from build123d import *
from build123d.topology import SkipClean

# Parameters (mm, degrees)
SKETCH2_W               = 173
SKETCH2_H               = 29.8
BOSS_EXTRUDE1_DEPTH     = 14
SKETCH4_W               = 173
SKETCH4_H               = 29.8
SKETCH4_R               = 1
BOSS_EXTRUDE3_DEPTH     = 2
BOSS_EXTRUDE4_START     = 5.5
SKETCH5_R               = 1
BOSS_EXTRUDE4_DEPTH     = 5.5
CUT_EXTRUDE1_DEPTH      = 91.874033815
CUT_EXTRUDE1_DEPTH_BACK = 91.874033815


with BuildPart() as part:
    # Sketch2 → Boss-Extrude1 (new body)
    with BuildSketch(Plane(origin=(0, 0, 0), x_dir=(1, 0, 0), z_dir=(0, 1, 0))):
        with Locations((0, 7.9)):
            Rectangle(SKETCH2_W, SKETCH2_H)
        with BuildLine():
            Line((-81.5, 0), (81.5, 0))
            add(Edge.make_bspline(
                [(-81.5, 0), (-74.436091259, 13.881927863), (-43.259356961, 16.362188276), (0, 18.555927536), (43.259356961, 16.362188276), (74.436091259, 13.881927863), (81.5, 0)],
                knots=[0, 0, 0, 0, 0.237125688, 0.5, 0.762874312, 1, 1, 1, 1], degree=3))
        make_face(mode=Mode.SUBTRACT)
    extrude(amount=BOSS_EXTRUDE1_DEPTH)

    # Sketch4 → Boss-Extrude3 (add)
    with BuildSketch(Plane(origin=(0, 14, 0), x_dir=(1, 0, 0), z_dir=(0, 1, 0))):
        with Locations((0, 7.9)):
            Rectangle(SKETCH4_W, SKETCH4_H)
        with Locations(Location((0, 12.8, 0), (0, 0, 270))):
            Circle(SKETCH4_R, mode=Mode.SUBTRACT)
    extrude(amount=BOSS_EXTRUDE3_DEPTH)

    # Sketch5 → Boss-Extrude4 (add)
    with SkipClean():  # the faces are left unmerged after this step: merging them gives an invalid solid
        with BuildSketch(Plane.XZ.offset(-14).offset(BOSS_EXTRUDE4_START)):
            Polygon((0, -9.8), (-7.931348641, -17.731348641), (-7.931348641, -22.8), (7.931348641, -22.8), (7.931348641, -17.731348641), align=None)
            with Locations(Location((0, -12.8, 0), (0, 0, 270))):
                Circle(SKETCH5_R, mode=Mode.SUBTRACT)
        extrude(amount=-BOSS_EXTRUDE4_DEPTH)

    # Sketch3 → Cut-Extrude1 (cut, two sides: drawn at the far end of the back side and taken through both)
    with SkipClean():  # the faces are left unmerged after this step: merging them gives an invalid solid
        with BuildSketch(Plane(origin=(0, 0, 0), x_dir=(0, 0, -1), z_dir=(1, 0, 0)).offset(-CUT_EXTRUDE1_DEPTH_BACK)):
            Polygon((-48.86878806, -37), (4.996225752, 22.823158451), (1.280501625, 26.168811483), (-52.584512187, -33.654346968), align=None)
        extrude(amount=CUT_EXTRUDE1_DEPTH + CUT_EXTRUDE1_DEPTH_BACK, mode=Mode.SUBTRACT)


solid = part.part
Work out the finished part from the listing and answer in its coordinate system (mm). A direction names the side the tool comes from. Give positions to 0.01 mm unless a question says otherwise; leave off trailing zeros. One line per item, written item: value. Start each with the question number.
1. Find section A-A (y = 11). State how many separate pieces and enclosed holes the cut face has, then the cut area to 3 significant figures.
2. Consider probe 1 along Z at (x, y) = (0, 2); probe 2 along X at (y, z) = (15.35, -12.8); probe 3 along Z at (x, y) = (28.5, 8.5). Determine where each line is inside the solid, lowest interval first.
3. Given pin 1 (6 mm diameter, centred on x = -18.5, y = 13, fed in from +Z); pin 2 (8 mm diameter, centred on x = -55.5, z = -5, fed in from -Y); pin 3 (4 mm diameter, centred on x = 53, z = 2, fed in from +Y), each flat-ended and moving along its own axis, determine where each tip first touches the part or whether it passes through.
4. For faces 5 (the flat face through (-1, 16, -11)), 6 (the flat face through (-3.9, 11.2, -13.7)), determine the directions among +Z, -Z, +X, -X, +Y, -Y from which every point of the face is accessible in a straight line to the end or side of a thin tool.
5. For a pull along Z with two mould halves and no side action, classify faces 1 (the flat face through (-86.5, 8, -8)), 2 (the flat face through (4, 11.2, -13.8)), 3 (the flat face through (0, 8.5, -16)), 4 (the flat face through (-1, 5, 7)) as +Z half, -Z half, draft (parallel to the pull), parting line (faces both ways), or undercut.
Geometry results:
1. separate pieces: 1
1. enclosed holes: 2
1. area: 2,550 mm2
2. probe 1: -22.8 to -17.8, 0 to 7
2. probe 2: -86.5 to -1, 1 to 86.5
2. probe 3: -22.8 to -17.01, 0 to 7
3. pin 1: z = 6.55
3. pin 2: y = 14
3. pin 3: y = 16
4. face 5: +Z, -Z, +X, -X, +Y
4. face 6: -Y
5. face 1: draft
5. face 2: undercut
5. face 3: undercut
5. face 4: +Z half
